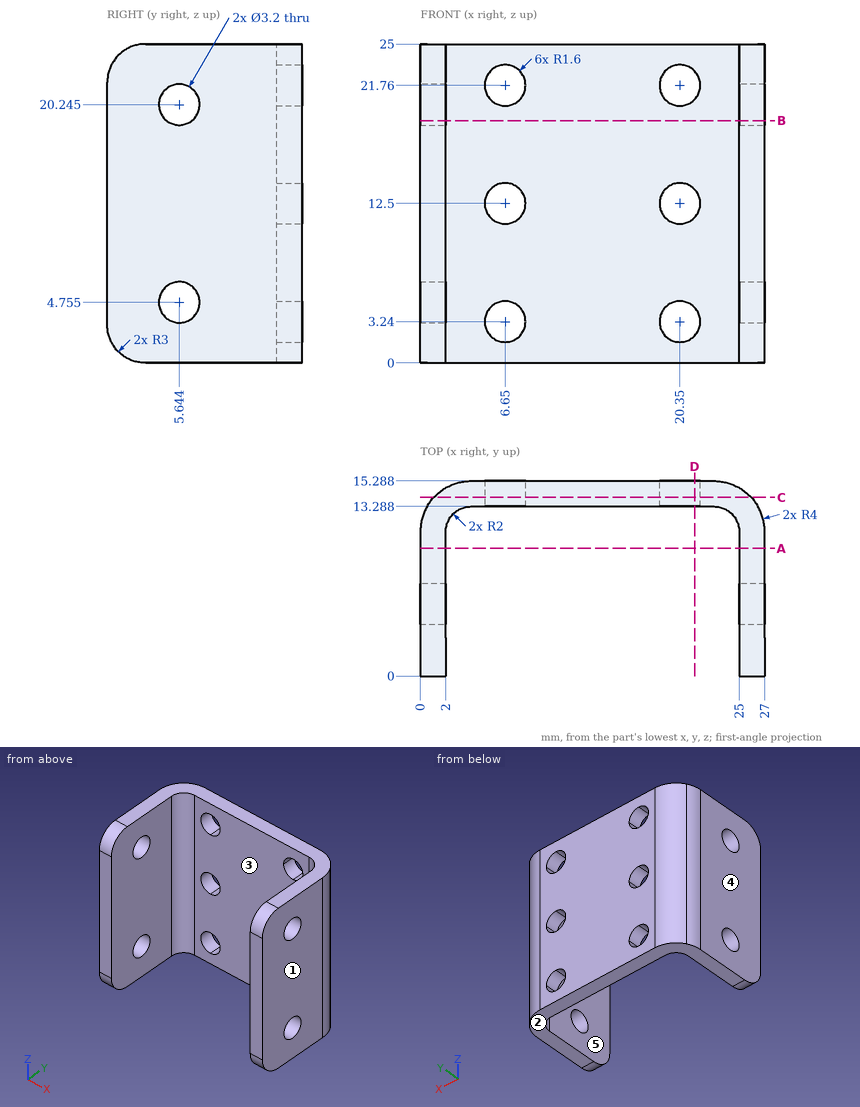
Can you work these out from the drawing? Everything is in mm from the part's minimum corner. A direction names the side the tool comes from. Coordinates: 2 decimals unless noted, no trailing zeros. Loops run counter-clockwise (first coordinate to the right, second up) from the corner with the lowest first, then second, coordinate; pieces in that order, holes last. Notation, with made-up numbers: M 23,43 L 33,43 A16 cw 33,53 Z; hole C -39,-26.5 d6. An arc over 180 degrees is marked long. One line per item, written item: value.
1. Imagine slicing it at A-A (y = 10). List the corners of the cut face in (x, z) for me.
Geometry says:
outline: M 0,0 L 2,0 L 2,25 L 0,25 Z; M 25,0 L 27,0 L 27,25 L 25,25 Z
2. On a 3-axis mill with a long thin cutter (end or side, diameter ignored), from which of +Z, -Z, +X, -X, +Y, -Y can I reach the whole of each face in a straight line? I mean the marked faces 4 and 5. Say none if no direction works.
Geometry says:
face 4: +Z, -Z, -X, +Y, -Y
face 5: +Z, -Z, -Y
3. Will these pins go through, and if not, where does the flat tip stop? pin 1 Ø1.5 at (x, z) = (3, 3.5) entering from -Y (1 decimal); pin 2 Ø3.5 at (y, z) = (5.64, 4.76) entering from +X; pin 3 Ø5.5 at (x, z) = (9, 15.5) entering from -Y.
Geometry says:
pin 1: stops at y = 12.3
pin 2: stops at x = 27
pin 3: stops at y = 13.29
4. Imagine slicing it at D-D (x = 21.5). List the corners of the cut face in (y, z) for me.
Geometry says:
outline: M 13.29,0 L 15.29,0 L 15.29,2.13 L 13.29,2.13 Z; M 13.29,4.35 L 15.29,4.35 L 15.29,11.39 L 13.29,11.39 Z; M 13.29,13.61 L 15.29,13.61 L 15.29,20.65 L 13.29,20.65 Z; M 13.29,22.87 L 15.29,22.87 L 15.29,25 L 13.29,25 Z
5. Imagine slicing it at B-B (z = 19). List the corners of the cut face in (x, y) for me.
Geometry says:
outline: M 0,0 L 2,0 L 2,4.64 L 0,4.64 Z; M 0,6.65 L 2,6.65 L 2,11.29 A2 cw 4,13.29 L 23,13.29 A2 cw 25,11.29 L 25,6.65 L 27,6.65 L 27,11.29 A4 ccw 23,15.29 L 4,15.29 A4 ccw 0,11.29 Z; M 25,0 L 27,0 L 27,4.64 L 25,4.64 Z
6. Thinking about a two-plate mould opening in X: for the marked faces 1, 2 and 3, which applies, +X half, -X half, draft (parallel to the pull), parting line (faces both ways), or undercut?
Geometry says:
face 1: +X half
face 2: draft
face 3: undercut
7. Imagine slicing it at C-C (y = 14). List the corners of the cut face in (x, z) for me, and give its area (3 significant figures).
Geometry says:
outline: M 1.06,0 L 25.94,0 L 25.94,25 L 1.06,25 Z; hole C 6.65,3.24 d3.2; hole C 6.65,12.5 d3.2; hole C 6.65,21.76 d3.2; hole C 20.35,3.24 d3.2; hole C 20.35,12.5 d3.2; hole C 20.35,21.76 d3.2
area: 574 mm2
8. Please list where these lines run through material, in increasing order: probe 1 along X at (y, z) = (7, 12.75); probe 2 along Y at (x, z) = (9, 21.5); probe 3 along X at (y, z) = (13, 10.5) (1 decimal).
Geometry says:
probe 1: x = 0 to 2, 25 to 27
probe 2: y = 13.29 to 15.29
probe 3: x = 0.4 to 3, 24 to 26.6
